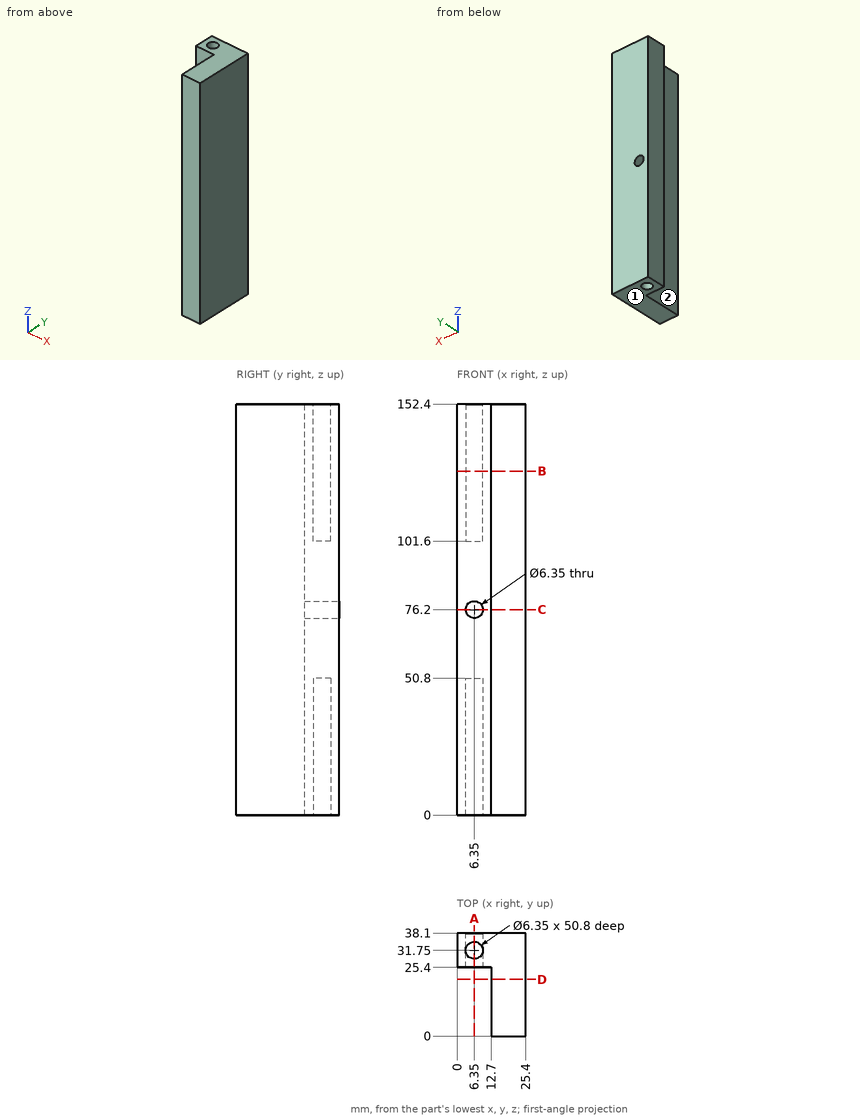
Could you check a few things on this drawing? It's one solid part, dimensions in mm from its lowest x, y, z. A direction names the side the tool comes from. Round coordinates to 2 decimals unless told otherwise and drop trailing zeros. Write each loop counter-clockwise with the first axis right and the second up, starting at its lowest first coordinate (ties: lowest second). Pieces come first, ordered by that corner, then holes. Notation, with made-up numbers: (29, 56) -> (68, 56) arc R22 ccw to (68, 62) -> close; hole circle Ø10 at (13, -27.75). An arc over 180 degrees is marked (long way). Use one line per item in the form item = value. Start each with the question number.
Q1. Which directions (+Z, -Z, +X, -X, +Y, -Y) give clear straight access to the entire face, cutting with the end or side of a thin tool? Please do the marked faces 1 and 2.
Q2. Imagine slicing it at A-A (x = 6.35). Please give me the cut outline in (y, z) (3 decimals), then the cut area to 3 significant figures.
Q3. Imagine slicing it at D-D (y = 21). Please give me the cut outline in (x, z), then the cut area to 3 significant figures.
Q4. Imagine slicing it at C-C (z = 76.2). Please give me the cut outline in (x, y) (3 decimals).
Q5. I'm going to push flat-ended pins straight in: P1, Ø14, axis at x = 7, z = 64.5, coming from the -Y side; P2, Ø10, axis at x = 6.35, z = 76.2, coming from the -Y side; P3, Ø5, axis at x = 6.35, y = 31.75, coming from the +Z side; P4, Ø7.5, axis at y = 8, z = 49.5, coming from the -X side. Where does each tip first touch, or does it pass through?
Q6. If I drill on probe 1 along X at (y, z) = (32, 76); probe 2 along Y at (x, z) = (6.35, 35) (3 decimals); probe 3 along Z at (x, y) = (6.35, 29) (3 decimals), over which ranges is the centre line in solid material (lowest first)? Write a range as [from, to].
Q7. Imagine slicing it at B-B (z = 127.5). Please give me the cut outline in (x, y) (3 decimals).
Worked out:
q1.face_1 = -Z, +X, -X, +Y, -Y
q1.face_2 = +Z, -Z, -X, -Y
q2.outline = (25.4, 0) -> (28.575, 0) -> (28.575, 50.8) -> (34.925, 50.8) -> (34.925, 0) -> (38.1, 0) -> (38.1, 73.025) -> (25.4, 73.025) -> close; (25.4, 79.375) -> (38.1, 79.375) -> (38.1, 152.4) -> (34.925, 152.4) -> (34.925, 101.6) -> (28.575, 101.6) -> (28.575, 152.4) -> (25.4, 152.4) -> close
q2.area = 1,210 mm^2
q3.outline = (12.7, 0) -> (25.4, 0) -> (25.4, 152.4) -> (12.7, 152.4) -> close
q3.area = 1,940 mm^2
q4.outline = (0, 25.4) -> (3.175, 25.4) -> (3.175, 38.1) -> (0, 38.1) -> close; (9.525, 25.4) -> (12.7, 25.4) -> (12.7, 0) -> (25.4, 0) -> (25.4, 38.1) -> (9.525, 38.1) -> close
q5.P1 = 0
q5.P2 = 25.4
q5.P3 = 101.6
q5.P4 = 12.7
q6.probe_1 = [0, 3.18], [9.52, 25.4]
q6.probe_2 = [25.4, 28.575], [34.925, 38.1]
q6.probe_3 = [50.8, 73.025], [79.375, 101.6]
q7.outline = (0, 25.4) -> (12.7, 25.4) -> (12.7, 0) -> (25.4, 0) -> (25.4, 38.1) -> (0, 38.1) -> close; hole circle Ø6.35 at (6.35, 31.75)
